```python
from build123d import *

# Parameters (mm, degrees)
F1_DEPTH = 317.5
F2_R     = 9.9949
F3_DEPTH = 25.4
F4_R     = 1.5
F5_DEPTH = 25.4
F6_R     = 5.08


with BuildPart() as f1:
    # F0 (on Right) → F1 (new body, symmetric)
    with BuildSketch(Plane.YZ):
        with BuildLine():
            Line((31.75, 0), (-31.75, 0))
            ThreePointArc((-31.75, 0), (-33.995064, -0.929936), (-34.925, -3.175))
            Line((-34.925, -3.175), (-34.925, -114.3))
            Line((-34.925, -114.3), (-33.3375, -114.3))
            Line((-33.3375, -114.3), (-33.3375, -3.175))
            ThreePointArc((-33.3375, -3.175), (-32.872532, -2.052468), (-31.75, -1.5875))
            Line((-31.75, -1.5875), (31.75, -1.5875))
            ThreePointArc((31.75, -1.5875), (32.872532, -2.052468), (33.3375, -3.175))
            Line((33.3375, -3.175), (33.3375, -114.3))
            Line((33.3375, -114.3), (34.925, -114.3))
            Line((34.925, -114.3), (34.925, -3.175))
            ThreePointArc((34.925, -3.175), (33.995064, -0.929936), (31.75, 0))
        make_face()
    extrude(amount=F1_DEPTH, both=True)

    # F2 (on face) → F3 (cut)
    with BuildSketch(Plane.XZ.offset(34.925)):
        with Locations((-279.4, -33.3375)):
            Circle(F2_R)
        with Locations((-279.4, -84.1375)):
            Circle(F2_R)
        with Locations((-228.6, -33.3375)):
            Circle(F2_R)
        with Locations((-228.6, -84.1375)):
            Circle(F2_R)
        with Locations((-177.8, -33.3375)):
            Circle(F2_R)
        with Locations((-177.8, -84.1375)):
            Circle(F2_R)
        with Locations((-127, -33.3375)):
            Circle(F2_R)
        with Locations((-127, -84.1375)):
            Circle(F2_R)
        with Locations((-76.2, -33.3375)):
            Circle(F2_R)
        with Locations((-76.2, -84.1375)):
            Circle(F2_R)
        with Locations((-25.4, -33.3375)):
            Circle(F2_R)
        with Locations((-25.4, -84.1375)):
            Circle(F2_R)
        with Locations((25.4, -33.3375)):
            Circle(F2_R)
        with Locations((25.4, -84.1375)):
            Circle(F2_R)
        with Locations((76.2, -33.3375)):
            Circle(F2_R)
        with Locations((76.2, -84.1375)):
            Circle(F2_R)
        with Locations((127, -33.3375)):
            Circle(F2_R)
        with Locations((127, -84.1375)):
            Circle(F2_R)
        with Locations((177.8, -33.3375)):
            Circle(F2_R)
        with Locations((177.8, -84.1375)):
            Circle(F2_R)
        with Locations((228.6, -33.3375)):
            Circle(F2_R)
        with Locations((228.6, -84.1375)):
            Circle(F2_R)
        with Locations((279.4, -33.3375)):
            Circle(F2_R)
        with Locations((279.4, -84.1375)):
            Circle(F2_R)
    extrude(amount=-F3_DEPTH, mode=Mode.SUBTRACT)

    # F4 (on face) → F5 (cut)
    with BuildSketch(Plane(origin=(0, 34.925, 0), x_dir=(-1, 0, 0), z_dir=(0, 1, 0))):
        with Locations((-23, -15.7375)):
            Circle(F4_R)
        with Locations((-23, -101.7375)):
            Circle(F4_R)
        with Locations((23, -15.7375)):
            Circle(F4_R)
        with Locations((23, -101.7375)):
            Circle(F4_R)
        with Locations((226.2, -101.7375)):
            Circle(F4_R)
        with Locations((180.2, -101.7375)):
            Circle(F4_R)
        with Locations((226.2, -15.7375)):
            Circle(F4_R)
        with Locations((180.2, -15.7375)):
            Circle(F4_R)
        with Locations((-226.2, -15.7375)):
            Circle(F4_R)
        with Locations((-180.2, -15.7375)):
            Circle(F4_R)
        with Locations((-180.2, -101.7375)):
            Circle(F4_R)
        with Locations((-226.2, -101.7375)):
            Circle(F4_R)
    extrude(amount=-F5_DEPTH, mode=Mode.SUBTRACT)

    # F6
    f6_edges = [f1.edges().sort_by_distance(p)[0] for p in [
        (-317.5, -34.13125, -114.3),
        (-317.5, 34.13125, -114.3),
        (317.5, -34.13125, -114.3),
        (317.5, 34.13125, -114.3),
    ]]
    fillet(f6_edges, radius=F6_R)


solid = f1.part
```
Geometry check sheet. Reference: the model listing, model coordinates, mm. A direction names the side the tool comes from. Round coordinates to 2 decimals unless told otherwise and drop trailing zeros. Loops run counter-clockwise (first coordinate to the right, second up) from the corner with the lowest first, then second, coordinate; pieces in that order, holes last. Notation, with made-up numbers: M -20.5,74 L 21.5,74 A22 ccw 21.5,91 Z; hole C 51.5,64 d4. An arc over 180 degrees is marked long. Return JSON: item names as keys, results as strings. Group by question number.
(1) Mould release check, pull along Y, two halves, no side actions. Record for faces 3 (the face through (4, 33.338, -58)), 4 (the face through (4, 34.925, -60)), 5 (the face through (66.215, -34.142, -32.898)): pulls with the +Y half, pulls with the -Y half, needs draft (parallel to the pull), parting line crosses it, or undercut.
(2) Set-up check for faces 1 (the face through (288.933, -34.142, -81.135)), 2 (the face through (4, 0, 0)): record each of +Z, -Z, +X, -X, +Y, -Y from which the full face is reachable in a straight line by a thin tool's end or side.
(3) Section check C-C, the plane y = -23. Enter the section's corners in (x, z).
(4) Section check A-A, the plane x = -279.4. Give the number of separate pieces and of enclosed holes in the cut face, and give its area (3 significant figures).
(5) Go/stop test with flat-tipped pins: pin 1 (5 mm diameter, centred on x = -226.2, z = -15.74, fed in from +Y) (3 decimals); pin 2 (12 mm diameter, centred on x = -279.4, z = -84.14, fed in from -Y); pin 3 (1.8 mm diameter, centred on x = 226.2, z = -15.74, fed in from +Y); pin 4 (5 mm diameter, centred on x = 165, y = 9.5, fed in from -Z). Record where each tip stops, or that it passes through.
(6) Scan lines: line 1 along Y through (x, z) = (-63, -104) (1 decimal); line 2 along Z through (x, y) = (76.2, -34.3); line 3 along Z through (x, y) = (127, -33.75). Record each from-to range of solid material in increasing order. Write a range as [from, to].
Data:
{
 "1": {"face 3": "undercut", "face 4": "pulls with the +Y half", "face 5": "needs draft"},
 "2": {"face 1": "-Y", "face 2": "+Z, +X, -X, +Y, -Y"},
 "3": {"outline": "M -317.5,-1.59 L 317.5,-1.59 L 317.5,0 L -317.5,0 Z"},
 "4": {"separate pieces": "3", "enclosed holes": "0", "area": "402 mm²"},
 "5": {"pin 1": "y = 34.925", "pin 2": "y = 33.34", "pin 3": "y = -33.34", "pin 4": "z = -1.59"},
 "6": {"line 1": "[-34.9, -33.3], [33.3, 34.9]", "line 2": "[-114.3, -94.13], [-74.14, -43.33], [-23.34, -1.28]", "line 3": "[-114.3, -94.13], [-74.14, -43.33], [-23.34, -0.71]"}
}
